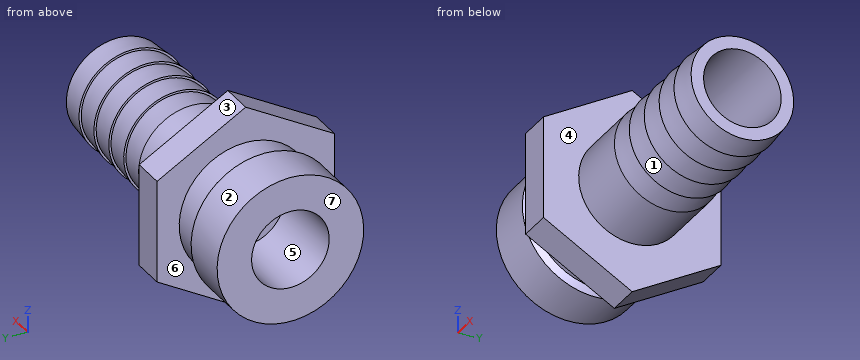
from build123d import *

# Parameters (mm, degrees)
LINEAR_AUSTRAGEN1_DEPTH = 6


with BuildPart() as part:
    # Skizze2 → Rotation1 (revolve)
    with BuildSketch(Plane.XY, mode=Mode.PRIVATE) as rotation1_sk:
        Polygon((5, 13.22), (5, 9.65), (21, 9.65), (23, 9.65), (28, 9.25), (28, 9.65), (33, 9.25), (33, 9.65), (38, 9.25), (38, 9.65), (43, 9.25), (43, 9.65), (48, 9.25), (48, 7), (-10, 7), (-10, 13.22), align=None)
    revolve(rotation1_sk.sketch.rotate(Axis((-12.825745381, 0, 0), (1, 0, 0)), 90), axis=Axis((-12.825745381, 0, 0), (1, 0, 0)))

    # Skizze4 → Linear austragen1 (add)
    with BuildSketch(Plane.ZY.offset(-5)):
        Polygon((9.237604307, -16), (18.475208614, 0), (9.237604307, 16), (-9.237604307, 16), (-18.475208614, 0), (-9.237604307, -16), align=None)
    extrude(amount=-LINEAR_AUSTRAGEN1_DEPTH)

    # Skizze5 → Schnitt-Rotation1 (revolve, cut)
    with BuildSketch(Plane.XY, mode=Mode.PRIVATE) as schnitt_rotation1_sk:
        Polygon((-2, 14.5), (-0.556624327, 12), (5, 12), (5, 14.5), align=None)
    revolve(schnitt_rotation1_sk.sketch.rotate(Axis((-12.825745381, 0, 0), (1, 0, 0)), 90), axis=Axis((-12.825745381, 0, 0), (1, 0, 0)), mode=Mode.SUBTRACT)


solid = part.part
Part model, mm, in its own coordinate system. Face numbers are marked on the shaded views. A direction names the side the tool comes from. Coordinates: 2 decimals unless noted, no trailing zeros. Write each loop counter-clockwise with the first axis right and the second up, starting at its lowest first coordinate (ties: lowest second). Pieces come first, ordered by that corner, then holes. Notation, with made-up numbers: (-38.75, 43) - (-11.75, 43) arc R20 cw to (-11.75, 77) - close; hole circle Ø2 at (39.5, 11.5). An arc over 180 degrees is marked (long way). Put each result on its own line as item: value.
1. Band-saw the part on A-A (x = 40). Write the cut outline in (y, z), then the cut area to 3 significant figures.
Final values:
outline: circle Ø18.98 at (0, 0); hole circle Ø14 at (0, 0)
area: 129 mm²
2. 3-axis set-ups, long thin cutter, end or side, ignore diameter. For the marked faces 1, 2, 3 and 4: which of +Z, -Z, +X, -X, +Y, -Y reach the whole face in a straight line?
Final values:
face 1: none
face 2: -X
face 3: +Z, +X, -X, +Y
face 4: +X
3. Band-saw the part on B-B (x = 6). Write the cut outline in (y, z).
Final values:
outline: (-16, -9.24) - (0, -18.48) - (16, -9.24) - (16, 9.24) - (0, 18.48) - (-16, 9.24) - close
4. Probe line 1 along Y through (x, z) = (-5, 0); line 2 along Y through (x, z) = (1.25, 0); line 3 along X through (y, z) = (-9, 10). List the from-to ranges inside material, lowest first. Write a range as [from, to].
Final values:
line 1: y = [-13.22, -7], [7, 13.22]
line 2: y = [-12, -7], [7, 12]
line 3: x = [5, 11]
5. Flat gauge pins, fed straight in: pin 1 Ø11 at (y, z) = (0, 0) entering from +X; pin 2 Ø6 at (y, z) = (-1, 0.5) entering from -X; pin 3 Ø1 at (x, y) = (33.5, 4.5) entering from -Z. Where does each tip first touch, or does it go through?
Final values:
pin 1: stops at x = 11
pin 2: stops at x = 5
pin 3: stops at z = -8.74
6. Two-plate mould, pull along X, no slides. Class the marked faces 5, 6 and 7: +X half, -X half, draft (parallel to the pull), parting line (faces both ways), or undercut.
Final values:
face 5: draft
face 6: undercut
face 7: -X half
